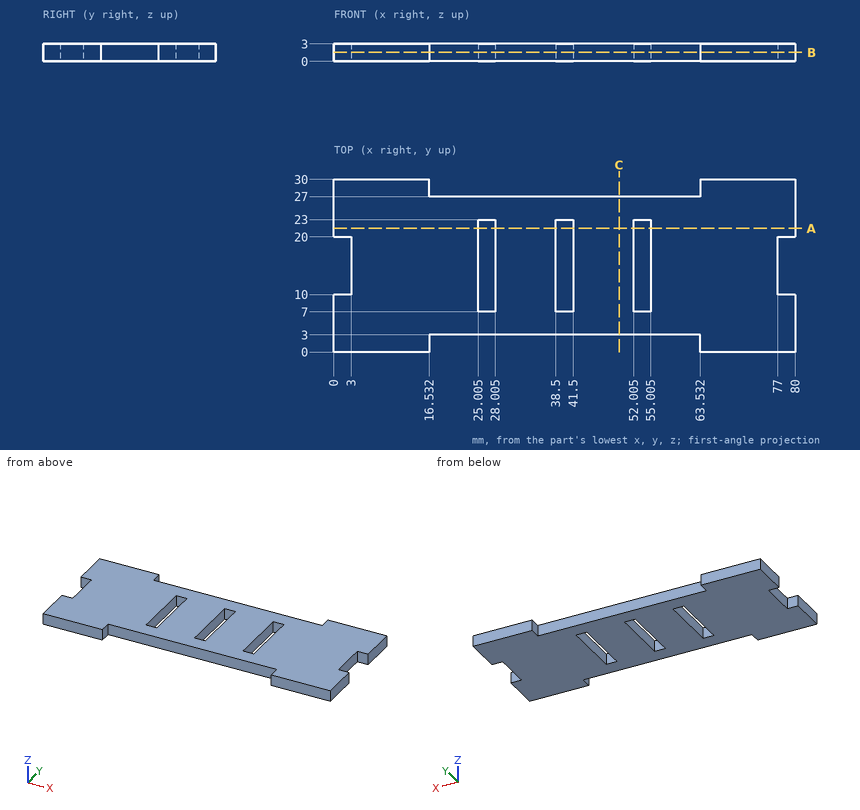
Study the drawing (mm; zero at the part's minimum x, y, z) and answer. Round coordinates to 2 decimals unless told otherwise and drop trailing zeros. Write each loop counter-clockwise with the first axis right and the second up, starting at its lowest first coordinate (ties: lowest second). Pieces come first, ordered by that corner, then holes. Notation, with made-up numbers: (55, 60) -> (69, 60) arc R25 cw to (69, 98) -> close; hole circle Ø10 at (37.25, 51.5). An arc over 180 degrees is marked (long way). Write item = value, one per line.
1) Given pin 1 (1.5 mm diameter, centred on x = 46, z = 2.5, fed in from -Y); pin 2 (0.9 mm diameter, centred on x = 42, z = 2, fed in from +Y), each flat-ended and moving along its own axis, determine where each tip first touches the part or whether it passes through.
Check values:
pin_1 = 3
pin_2 = 27
2) Section A-A on y = 21.5 is taken. Write down the section's boundary in (x, z) (1 decimal), plus the area to 3 significant figures.
Check values:
outline = (0, 0) -> (25, 0) -> (25, 3) -> (0, 3) -> close; (28, 0) -> (38.5, 0) -> (38.5, 3) -> (28, 3) -> close; (41.5, 0) -> (52, 0) -> (52, 3) -> (41.5, 3) -> close; (55, 0) -> (80, 0) -> (80, 3) -> (55, 3) -> close
area = 213 mm²
3) Section B-B on z = 1.55 is taken. Give the number of separate pieces and of enclosed holes in the cut face, plus the area to 3 significant figures.
Check values:
separate_pieces = 1
enclosed_holes = 3
area = 1,910 mm²
4) Straight lines are drawn through the part: line 1 along X through (y, z) = (12, 1.15) (1 decimal); line 2 along X through (y, z) = (9.25, 1.3) (1 decimal); line 3 along X through (y, z) = (2.75, 2.3). For each, find the intervals that lie inside material, in ascending order. Write a range as [from, to].
Check values:
line_1 = [3, 25], [28, 38.5], [41.5, 52], [55, 77]
line_2 = [0, 25], [28, 38.5], [41.5, 52], [55, 80]
line_3 = [0, 16.53], [63.53, 80]
5) Section C-C on x = 49.5 is taken. Write down the section's boundary in (y, z).
Check values:
outline = (3, 0) -> (27, 0) -> (27, 3) -> (3, 3) -> close
